CAD build for the part. Positions are in the model's coordinates, mm. Face numbers are marked on the shaded views. Round coordinates to 2 decimals unless told otherwise and drop trailing zeros. Loops run counter-clockwise (first coordinate to the right, second up) from the corner with the lowest first, then second, coordinate; pieces in that order, holes last.
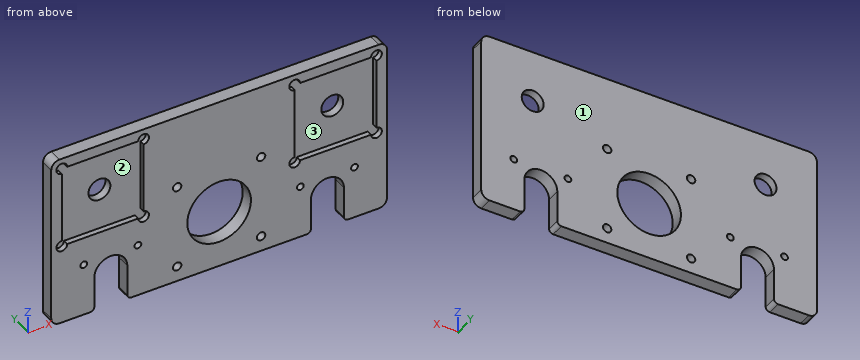
```python
from build123d import *

# Parameters (mm, degrees)
SKETCH1_W           = 124
SKETCH1_H           = 64
BOSS_EXTRUDE1_DEPTH = 5
CUT_EXTRUDE1_DEPTH  = 5
SKETCH3_W           = 30.202540726
SKETCH3_H           = 30.202540726
CUT_EXTRUDE2_DEPTH  = 2
SKETCH4_R           = 2
CUT_EXTRUDE3_DEPTH  = 2
SKETCH5_R           = 4.05
SKETCH5_R_2         = 1.55
SKETCH5_R_3         = 11.75
CUT_EXTRUDE4_DEPTH  = 5
SKETCH6_R           = 1.25
CUT_EXTRUDE5_DEPTH  = 10
FILLET1_R           = 3
FILLET2_R           = 1.5


with BuildPart() as part:
    # Sketch1 → Boss-Extrude1 (new body)
    with BuildSketch(Plane(origin=(0, 0, 0), x_dir=(1, 0, 0), z_dir=(0, 1, 0))):
        with Locations((62, -32)):
            Rectangle(SKETCH1_W, SKETCH1_H)
    extrude(amount=BOSS_EXTRUDE1_DEPTH)

    # Sketch2 → Cut-Extrude1 (cut)
    with BuildSketch(Plane(origin=(0, 5, 0), x_dir=(1, 0, 0), z_dir=(0, 1, 0))):
        with BuildLine():
            Line((15.897459274, -12.997459274), (15.897459274, 12.365379101))
            Line((15.897459274, 12.365379101), (28.097459274, 12.365379101))
            Line((28.097459274, 12.365379101), (28.097459274, -12.997459274))
            ThreePointArc((28.097459274, -12.997459274), (21.997459274, -19.097459274), (15.897459274, -12.997459274))
        make_face()
        with BuildLine():
            Line((95.902540726, 12.365379101), (95.902540726, -12.997459274))
            ThreePointArc((95.902540726, -12.997459274), (102.002540726, -19.097459274), (108.102540726, -12.997459274))
            Line((108.102540726, -12.997459274), (108.102540726, 12.365379101))
            Line((108.102540726, 12.365379101), (95.902540726, 12.365379101))
        make_face()
    extrude(amount=-CUT_EXTRUDE1_DEPTH, mode=Mode.SUBTRACT)

    # Sketch3 → Cut-Extrude2 (cut)
    with BuildSketch(Plane.XZ):
        with Locations((18.998729637, 44.998729637)):
            Rectangle(SKETCH3_W, SKETCH3_H)
        with Locations((105.001270363, 44.998729637)):
            Rectangle(SKETCH3_W, SKETCH3_H)
    extrude(amount=-CUT_EXTRUDE2_DEPTH, mode=Mode.SUBTRACT)

    # Sketch4 → Cut-Extrude3 (cut)
    with BuildSketch(Plane.XZ):
        with Locations((34.1, 29.897459274)):
            Circle(SKETCH4_R)
        with Locations((34.1, 60.1)):
            Circle(SKETCH4_R)
        with Locations((3.897459274, 60.1)):
            Circle(SKETCH4_R)
        with Locations((3.897459274, 29.897459274)):
            Circle(SKETCH4_R)
        with Locations((120.102540726, 29.897459274)):
            Circle(SKETCH4_R)
        with Locations((120.102540726, 60.1)):
            Circle(SKETCH4_R)
        with Locations((89.9, 60.1)):
            Circle(SKETCH4_R)
        with Locations((89.9, 29.897459274)):
            Circle(SKETCH4_R)
    extrude(amount=-CUT_EXTRUDE3_DEPTH, mode=Mode.SUBTRACT)

    # Sketch5 → Cut-Extrude4 (cut)
    with BuildSketch(Plane.XZ):
        with Locations(Location((18.998729637, 44.998729637, 0), (0, 0, 270))):
            Circle(SKETCH5_R)
        with Locations(Location((105.001270363, 44.998729637, 0), (0, 0, 270))):
            Circle(SKETCH5_R)
        with Locations(Location((77.5, 36.648702719, 0), (0, 0, 270))):
            Circle(SKETCH5_R_2)
        with Locations(Location((46.5, 36.648702719, 0), (0, 0, 270))):
            Circle(SKETCH5_R_2)
        with Locations(Location((46.5, 5.648702719, 0), (0, 0, 270))):
            Circle(SKETCH5_R_2)
        with Locations(Location((77.5, 5.648702719, 0), (0, 0, 270))):
            Circle(SKETCH5_R_2)
        with Locations(Location((62, 21.148702719, 0), (0, 0, 270))):
            Circle(SKETCH5_R_3)
    extrude(amount=-CUT_EXTRUDE4_DEPTH, mode=Mode.SUBTRACT)

    # Sketch6 → Cut-Extrude5 (cut)
    with BuildSketch(Plane(origin=(0, 5, 0), x_dir=(1, 0, 0), z_dir=(0, 1, 0))):
        with Locations(Location((11.997459274, -19.497459274, 0), (0, 0, 270))):
            Circle(SKETCH6_R)
        with Locations(Location((31.997459274, -19.497459274, 0), (0, 0, 270))):
            Circle(SKETCH6_R)
        with Locations(Location((92.002540726, -19.497459274, 0), (0, 0, 270))):
            Circle(SKETCH6_R)
        with Locations(Location((112.002540726, -19.497459274, 0), (0, 0, 270))):
            Circle(SKETCH6_R)
    extrude(amount=-CUT_EXTRUDE5_DEPTH, mode=Mode.SUBTRACT)

    # Fillet1
    fillet1_edges = [part.edges().sort_by_distance(p)[0] for p in [
        (0, 2.5, 0),
        (124, 2.5, 0),
        (124, 2.5, 64),
        (0, 2.5, 64),
    ]]
    fillet(fillet1_edges, radius=FILLET1_R)

    # Fillet2
    fillet2_edges = [part.edges().sort_by_distance(p)[0] for p in [
        (15.897459274, 2.5, 0),
        (28.097459274, 2.5, 0),
        (95.902540726, 2.5, 0),
        (108.102540726, 2.5, 0),
    ]]
    fillet(fillet2_edges, radius=FILLET2_R)


solid = part.part
```
Item 1: Probe line 1 (Z direction, x = 77.5, y = 2.9); line 2 (X direction, y = 1.5, z = 33); line 3 (Z direction, x = 35.5, y = 0.35). List the from-to ranges inside material, lowest first.
Answers follow:
line 1: z = 0 to 4.1, 7.2 to 35.1, 38.2 to 64
line 2: x = 0 to 3.9, 34.1 to 89.9, 120.1 to 124
line 3: z = 0 to 28.47, 31.33 to 58.67, 61.53 to 64
Item 2: Flat gauge pins, fed straight in: P1, Ø10.5, axis at x = 12.5, z = 40.5, coming from the -Y side; P2, Ø12, axis at x = 105.5, z = 48, coming from the +Y side; P3, Ø1.5, axis at x = 17.5, y = 2, coming from the -Z side. Where does each tip first touch, or does it go through?
Answers follow:
P1: stops at y = 2
P2: stops at y = 5
P3: stops at z = 16.11
Item 3: Cut at B-B, the plane x = 46.5. Give the cut face in (y, z), plus the area to 3 significant figures.
Answers follow:
outline: (0, 0) - (5, 0) - (5, 4.1) - (0, 4.1) - close; (0, 7.2) - (5, 7.2) - (5, 35.1) - (0, 35.1) - close; (0, 38.2) - (5, 38.2) - (5, 64) - (0, 64) - close
area: 289 mm2
Item 4: Two-plate mould, pull along Z, no slides. Class the marked faces 1, 2 and 3: released by +Z, released by -Z, zero draft, split by the parting line, or undercut.
Answers follow:
face 1: zero draft
face 2: undercut
face 3: undercut
Item 5: Cut at D-D, the plane y = 3.9. State how many separate pieces and enclosed holes the cut face has, plus the area to 3 significant figures.
Answers follow:
separate pieces: 1
enclosed holes: 11
area: 6,910 mm2
Item 6: Cut at C-C, the plane z = 25.5. Give the cut face in (x, y).
Answers follow:
outline: (0, 0) - (51.09, 0) - (51.09, 5) - (0, 5) - close; (72.91, 0) - (124, 0) - (124, 5) - (72.91, 5) - close
Item 7: Cut at A-A, the plane x = 62. Give the cut face in (y, z).
Answers follow:
outline: (0, 0) - (5, 0) - (5, 9.4) - (0, 9.4) - close; (0, 32.9) - (5, 32.9) - (5, 64) - (0, 64) - close
